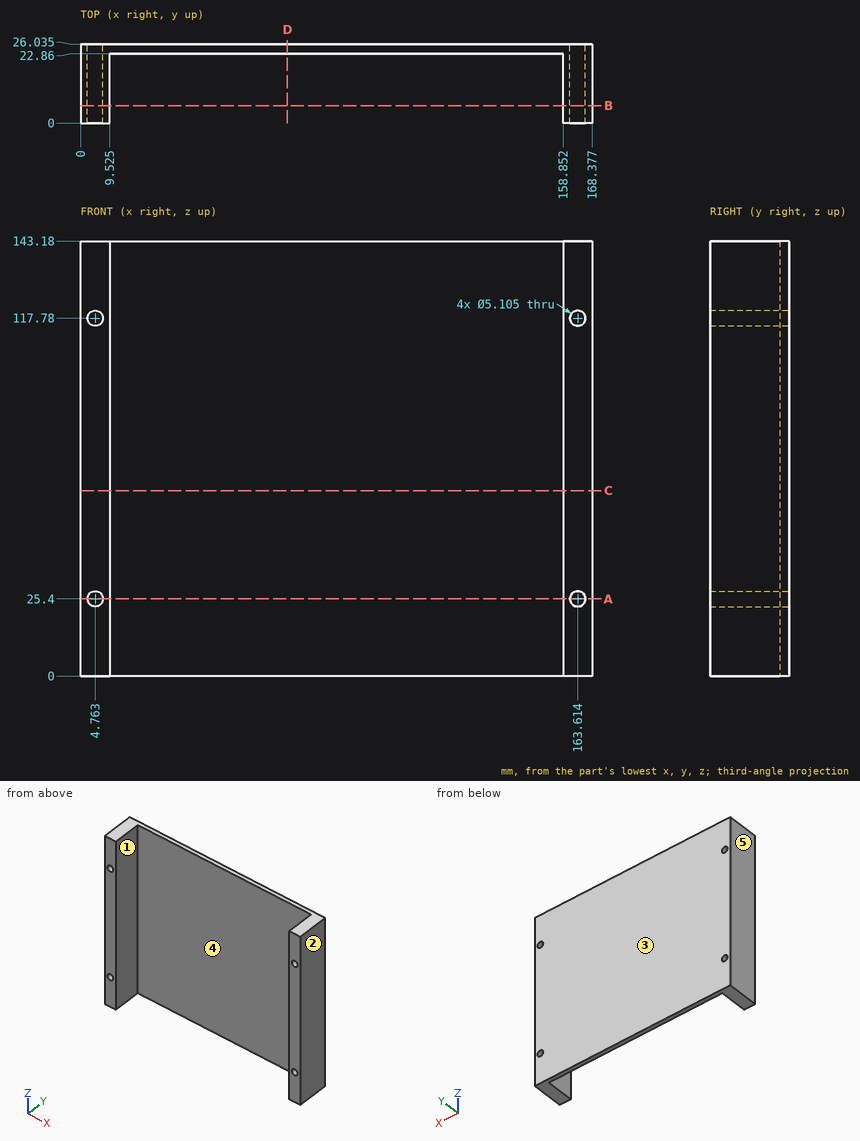
For this review, use the dimensioned drawing (mm, ordinates from the lowest corner) and the shaded views. A direction names the side the tool comes from. Coordinates: 2 decimals unless noted, no trailing zeros. Write each loop counter-clockwise with the first axis right and the second up, starting at its lowest first coordinate (ties: lowest second). Pieces come first, ordered by that corner, then holes. Notation, with made-up numbers: (46.25, -24) -> (72.25, -24) arc R10 ccw to (72.25, -8) -> close; hole circle Ø4 at (36, -30). An arc over 180 degrees is marked (long way). Write each question's results on one line, items separated by ' | '. Start each with the question number.
(1) Take a section at A-A on z = 25.4. Write out the cut boundary in (x, y) (1 decimal).
(2) For line 1 along X through (y, z) = (20.75, 25.4) (1 decimal); line 2 along X through (y, z) = (10.25, 34.5) (1 decimal); line 3 along Z through (x, y) = (161.5, 16.5), list the stretches that pass through material, from the lowest coordinate up. Write a range as from..to.
(3) Take a section at C-C on z = 61. Write out the cut boundary in (x, y) (1 decimal).
(4) The part is to be moulded in two halves that separate along X. For the marked faces 3, 4 and 5, say which applies: pulls with the +X half, pulls with the -X half, needs draft (parallel to the pull), parting line crosses it, or undercut.
(5) Take a section at B-B on y = 5.75. Write out the cut boundary in (x, z) (1 decimal), and give its area (3 significant figures).
(6) Tool access review of the marked faces 1 and 2: name each direction out of +Z, -Z, +X, -X, +Y, -Y from which nothing blocks a thin tool from reaching the whole face with its end or side.
(7) Take a section at D-D on x = 68. Write out the cut boundary in (y, z) (1 decimal).
(8) Clearance check with a flat-ended pin moving along its axis: P1, Ø6, axis at x = 118, z = 41.5, coming from the -Y side. State where the tip first meets the part, or that it passes through.
Results found:
1) outline: (0, 0) -> (2.2, 0) -> (2.2, 26) -> (0, 26) -> close; (7.3, 0) -> (9.5, 0) -> (9.5, 22.9) -> (158.9, 22.9) -> (158.9, 0) -> (161.1, 0) -> (161.1, 26) -> (7.3, 26) -> close; (166.2, 0) -> (168.4, 0) -> (168.4, 26) -> (166.2, 26) -> close
2) line 1: x = 0..2.2, 7.3..9.5, 158.9..161.1, 166.2..168.4 | line 2: x = 0..9.5, 158.9..168.4 | line 3: z = 0..23.97, 26.83..116.35, 119.21..143.18
3) outline: (0, 0) -> (9.5, 0) -> (9.5, 22.9) -> (158.9, 22.9) -> (158.9, 0) -> (168.4, 0) -> (168.4, 26) -> (0, 26) -> close
4) face 3: needs draft | face 4: undercut | face 5: pulls with the -X half
5) outline: (0, 0) -> (9.5, 0) -> (9.5, 143.2) -> (0, 143.2) -> close; (158.9, 0) -> (168.4, 0) -> (168.4, 143.2) -> (158.9, 143.2) -> close; hole circle Ø5.1 at (4.8, 25.4); hole circle Ø5.1 at (4.8, 117.8); hole circle Ø5.1 at (163.6, 25.4); hole circle Ø5.1 at (163.6, 117.8) | area: 2,650 mm2
6) face 1: +Z, -Z, -Y | face 2: +Z, -Z, +X, +Y, -Y
7) outline: (22.9, 0) -> (26, 0) -> (26, 143.2) -> (22.9, 143.2) -> close
8) P1: stops at y = 22.86
